Autodesk Inventor part; units mm, degrees
ref_plane "Work Plane1" through (0, 0, 4950) normal (0, 0, 1) x (1, 0, 0)
ref_plane "Work Plane2" through (0, 0, 4954) normal (0, 0, 1) x (1, 0, 0)
ref_plane "Work Plane3" through (-40, 73, 4950) normal (0, -1, 0) x (1, 0, 0)
ref_plane "Work Plane1" through (0, 0, 4950) normal (0, 0, 1) x (1, 0, 0)
sketch "Sketch1" plane through (0, 0, 4950) normal (0, 0, 1) x (1, 0, 0)
  circle A0 centre (180, 0) radius 12.5
  circle A1 centre (180, 17.5) radius 2
  circle A2 centre (197.5, 0) radius 2
  circle A3 centre (162.5, 0) radius 2
  circle A4 centre (180, -17.5) radius 2
  line L0 (40, 182.7) -> (-40, 182.7)
  line L1 (-40, 182.7) -> (-40, -182.7)
  line L2 (-40, -182.7) -> (40, -182.7)
  line L3 (40, -182.7) -> (40, -50)
  line L4 (40, -50) -> (260, -50)
  line L5 (260, -50) -> (260, 50)
  line L6 (260, 50) -> (40, 50)
  line L7 (40, 50) -> (40, 182.7)
  circle A5 centre (0, 120) radius 8
  circle A6 centre (0, -120) radius 8
  circle A7 centre (0, -120) radius 8.5
  circle A8 centre (0, 120) radius 8.5
  line L8 (40, 182.7) -> (40, -182.7)
  line L9 (40, -182.7) -> (80, -182.7)
  line L10 (80, -182.7) -> (80, 182.7)
  line L11 (80, 182.7) -> (40, 182.7)
  line L12 (-40, 75) -> (40, 75)
  line L13 (40, 75) -> (40, -75)
  line L14 (40, -75) -> (-40, -75)
  line L15 (80, 182.7) -> (260, 50)
  line L16 (260, -50) -> (80, -182.7)
  line L17 (80, -142.7) -> (-40, -142.7)
  line L18 (-40, 142.7) -> (80, 142.7)
  line L19 (80, 142.7) -> (134.2577, 142.7)
  line L20 (80, -142.7) -> (134.2577, -142.7)
  line L21 (210, 86.8611) -> (210, -86.8611)
  point P0 (0, 0)
  point P1 (40, 75)
  dimension "d0" = 17
  dimension "d1" = 17
  dimension "d2" = 40
  dimension "d3" = 40
  dimension "d4" = 75
  dimension "d5" = 75
  dimension "d23" = 40
  dimension "d24" = 40
  dimension "d25" = 50
extrude "Extrusion1" add sketch "Sketch1" along normal blind 8 contours A0 | A1 | A2 | A3 | A4 | L18 L10 L6 L7 | L7 L12 L1 L18 | L19 L15 L21 L6 L10 | L6 L10 L4 L8 | L6 L21 L4 L10 | L14 L3 L17 L1 | L4 L10 L17 L3 | L4 L21 L16 L20 L10
sketch "Sketch2" plane through (0, 0, 4958) normal (0, 0, 1) x (1, 0, 0)
  line L0 (-40, 75) -> (40, 75)
  line L1 (-40, 75) -> (40, 75)
  line L2 (40, 75) -> (40, 79)
  line L3 (40, 79) -> (-40, 79)
  line L4 (-40, 79) -> (-40, 75)
  line L5 (40, -75) -> (-40, -75)
  line L6 (40, -75) -> (-40, -75)
  line L7 (-40, -75) -> (-40, -79)
  line L8 (-40, -79) -> (40, -79)
  line L9 (40, -79) -> (40, -75)
  line L10 (-20, 79) -> (-20, -79)
  line L11 (20, -79) -> (20, 79)
  point P0 (0, 0)
  point P1 (20, 75)
  point P2 (-20, 75)
  point P3 (20, -75)
  point P4 (-20, -75)
  dimension "d8" = 4
  dimension "d9" = 4
  dimension "d12" = 20
  dimension "d13" = 20
extrude "Extrusion2" add sketch "Sketch2" along normal blind 50 contours L10 L3 L11 L0 | L5 L11 L8 L10
sketch "Sketch3" plane through (-40, -75, 4950) normal (0, 1, 0) x (1, 0, 0)
  circle A0 centre (40, -38) radius 10.5
  line L0 (60, -58) -> (20, -58)
  line L1 (20, -8) -> (20, -58)
  point P0 (40, 4950)
  dimension "d16" = 21
  dimension "d17" = 20
  dimension "d18" = 20
extrude "Extrusion3" add sketch "Sketch3" along normal blind 163 and the other way blind 13
sketch "Sketch4" plane through (0, 0, 4958) normal (0, 0, 1) x (1, 0, 0)
  circle A0 centre (160, 17.5) radius 2
  circle A1 centre (177.5, 0) radius 2
  circle A2 centre (0, -120) radius 8
  circle A3 centre (142.5, 0) radius 2
  circle A4 centre (160, -17.5) radius 2
  circle A5 centre (0, 120) radius 8
  line L0 (30, 157.3) -> (30, 182.7)
  line L1 (40, 182.7) -> (30, 182.7)
  line L2 (40, 50) -> (40, 182.7)
  line L3 (260, 50) -> (40, 50)
  line L4 (260, -50) -> (260, 50)
  line L5 (40, -50) -> (260, -50)
  line L6 (40, -182.7) -> (40, -50)
  line L7 (30, -182.7) -> (40, -182.7)
  line L8 (30, -182.7) -> (30, -157.3)
  line L9 (30, -157.3) -> (-30, -157.3)
  line L10 (-30, -157.3) -> (-30, -182.7)
  line L11 (-40, -182.7) -> (-30, -182.7)
  line L12 (-40, 182.7) -> (-40, -182.7)
  line L13 (-30, 182.7) -> (-40, 182.7)
  line L14 (-30, 182.7) -> (-30, 157.3)
  line L15 (-30, 157.3) -> (30, 157.3)
  line L16 (250, 25.4) -> (224.6, 25.4)
  line L17 (224.6, 25.4) -> (224.6, -25.4)
  line L18 (224.6, -25.4) -> (250, -25.4)
  line L19 (250, -25.4) -> (250, 25.4)
  circle A6 centre (160, 0) radius 10
  point P0 (0, 0)
extrude "Extrusion4" cut sketch "Sketch4" against normal up to surface (8 mm away) contours A0 | A1 | A3 | A4
sketch "Sketch5" plane through (0, 0, 4958) normal (0, 0, 1) x (1, 0, 0)
  circle A0 centre (160, 0) radius 7.5
  circle A1 centre (160, 0) radius 8.25
  point P0 (0, 0)
  dimension "d28" = 16.5
extrude "Extrusion5" cut sketch "Sketch5" against normal blind 10 contours A0 | A1
sketch "Sketch6" plane through (0, 0, 4950) normal (0, 0, -1) x (-1, 0, 0)
  circle A0 centre (-142.5, 0) radius 2
  circle A1 centre (-177.5, 0) radius 2
  circle A2 centre (-160, 17.5) radius 2
  circle A3 centre (-160, -17.5) radius 2
  line L0 (-134.2577, 142.7) -> (40, 142.7)
  line L1 (-210, 86.8611) -> (-134.2577, 142.7)
  line L2 (-210, -86.8611) -> (-210, 86.8611)
  line L3 (-134.2577, -142.7) -> (-210, -86.8611)
  line L4 (40, -142.7) -> (-134.2577, -142.7)
  line L5 (40, -75) -> (40, -142.7)
  line L6 (-40, -75) -> (40, -75)
  line L7 (-40, 75) -> (-40, -75)
  line L8 (40, 75) -> (-40, 75)
  line L9 (40, 142.7) -> (40, 75)
  circle A4 centre (0, -120) radius 8.5
  circle A5 centre (0, 120) radius 8.5
  circle A6 centre (-160, 0) radius 8.25
  circle A7 centre (-160, 0) radius 22.5
  point P0 (0, 0)
  dimension "d31" = 45
extrude "Extrusion6" add sketch "Sketch6" along normal blind 4 contours A7
sketch "Sketch7" plane through (160, 0, 4946) normal (0, 0, -1) x (-1, 0, 0)
  circle A0 centre (0, 0) radius 22.5
  circle A1 centre (0, 0) radius 12.5
  circle A2 centre (0, 0) radius 9
  point P0 (160, 0)
  dimension "d34" = 25
  dimension "d47" = 18
extrude "Extrusion7" add sketch "Sketch7" along normal blind 40 contours A1
sketch "Sketch9" plane through (0, 0, 5008) normal (0, 0, 1) x (1, 0, 0)
  circle A0 centre (160, 0) radius 8.25 construction
  circle A1 centre (142.5, 0) radius 2 construction
  circle A2 centre (177.5, 0) radius 2 construction
  circle A3 centre (160, 17.5) radius 2 construction
  circle A4 centre (160, -17.5) radius 2 construction
  line L0 (20, 79) -> (20, 75)
  line L1 (20, 75) -> (40, 75)
  line L2 (40, 75) -> (40, -75)
  line L3 (40, -75) -> (20, -75)
  line L4 (20, -75) -> (20, -79)
  line L5 (20, -79) -> (-20, -79)
  line L6 (-20, -79) -> (-20, -75)
  line L7 (-20, -75) -> (-40, -75)
  line L8 (-40, -75) -> (-40, -142.7)
  line L9 (-40, -142.7) -> (134.2577, -142.7)
  line L10 (134.2577, -142.7) -> (210, -86.8611)
  line L11 (210, -86.8611) -> (210, 86.8611)
  line L12 (210, 86.8611) -> (134.2577, 142.7)
  line L13 (134.2577, 142.7) -> (-40, 142.7)
  line L14 (-40, 142.7) -> (-40, 75)
  line L15 (-40, 75) -> (-20, 75)
  line L16 (-20, 75) -> (-20, 79)
  line L17 (-20, 79) -> (20, 79)
  circle A5 centre (0, -120) radius 8.5
  circle A6 centre (0, 120) radius 8.5
  circle A7 centre (160, 0) radius 12.5
  circle A8 centre (160, 0) radius 9
  line L18 (20, -75) -> (-20, -75)
  line L19 (-20, 75) -> (20, 75)
  point P0 (0, 0)
  dimension "d37" = 18
extrude "Extrusion8" [suppressed]
sketch "Sketch10" plane through (0, 0, 5012) normal (0, 0, 1) x (1, 0, 0)
  circle A0 centre (120, -75) radius 6
  circle A1 centre (90, 0) radius 6
  circle A2 centre (120, 75) radius 6
  circle A3 centre (160, 0) radius 12.5
  point P0 (0, 0)
  dimension "d40" = 70
  dimension "d41" = 75
  dimension "d42" = 75
  dimension "d43" = 40
  dimension "d44" = 12
extrude "Extrusion9" [suppressed]
sketch "Sketch11" plane through (20, -79, 4958) normal (1, 0, 0) x (0, 0, -1)
  line L0 (0, 4) -> (0, 0)
  line L1 (0, 4) -> (-50, 4)
  line L2 (-50, 0) -> (-50, 4)
  line L3 (0, 0) -> (-50, 0)
  line L4 (0, 158) -> (0, 154)
  line L5 (0, 158) -> (-50, 158)
  line L6 (-50, 154) -> (-50, 158)
  line L7 (0, 154) -> (-50, 154)
  point P0 (4958, 79)
extrude "Extrusion10" add sketch "Sketch11" along normal blind 190
sketch "Sketch12" plane through (-20, -79, 4958) normal (-1, 0, 0) x (0, 0, 1)
  line L0 (0, 154) -> (0, 158)
  line L1 (0, 154) -> (50, 154)
  line L2 (50, 158) -> (50, 154)
  line L3 (0, 158) -> (50, 158)
  line L4 (0, 0) -> (0, 4)
  line L5 (0, 0) -> (50, 0)
  line L6 (50, 4) -> (50, 0)
  line L7 (0, 4) -> (50, 4)
  point P0 (-4958, 79)
extrude "Extrusion11" add sketch "Sketch12" along normal up to surface (20 mm away)
ref_plane "Work Plane2" through (0, 0, 4954) normal (0, 0, 1) x (1, 0, 0)
mirror "Mirror1" about plane through (0, 0, 4954) normal (0, 0, 1) of "Extrusion6", "Extrusion7"
sketch "Sketch13" plane through (160, 0, 4906) normal (0, 0, -1) x (-1, 0, 0)
  circle A0 centre (0, 0) radius 9
  circle A1 centre (4, 28) radius 75.6042
  point P0 (160, 0)
extrude "Extrusion12" cut sketch "Sketch13" against normal up to surface (44 mm away)
ref_plane "Work Plane3" through (-40, 73, 4950) normal (0, -1, 0) x (1, 0, 0)
sketch "Sketch14" plane through (-40, 73, 4950) normal (0, -1, 0) x (1, 0, 0)
  circle A0 centre (40, 38) radius 10.5
  line L0 (0, 8) -> (250, 8)
  line L1 (0, 8) -> (0, 58)
  line L2 (0, 58) -> (250, 58)
  line L3 (250, 8) -> (250, 58)
  circle A1 centre (40, 38) radius 12
  point P0 (40, -4950)
  dimension "d55" = 24
extrude "Extrusion13" add sketch "Sketch14" along normal blind 2 contours A1
mirror "Mirror2" about plane through (0, 0, 0) normal (0, 1, 0) of "Extrusion13"
ref_plane "Work Plane4" through (-40, 0, 4950) normal (0, 1, 0) x (1, 0, 0)
sketch "Sketch15" plane through (-40, 0, 4950) normal (0, 1, 0) x (1, 0, 0)
  circle A0 centre (40, -38) radius 10.5
  circle A1 centre (40, -38) radius 10.5
  circle A2 centre (40, -38) radius 17.5
  point P0 (40, 4950)
  dimension "d58" = 35
extrude "Extrusion14" add sketch "Sketch15" along normal mid plane 37
pattern_linear "Rectangular Pattern1" count 2 spacing 29 along (0, -1, 0) of "Extrusion13"
mirror "Mirror3" about plane through (0, 0, 0) normal (0, 1, 0) of "Extrusion13", "Rectangular Pattern1"
equation "\"d8\" = d9"
properties part number "base for ball scew -bolt" material "Steel, Mild"
Geometry check sheet. Reference: the model listing, model coordinates, mm. A direction names the side the tool comes from. Round coordinates to 2 decimals unless told otherwise and drop trailing zeros. Loops run counter-clockwise (first coordinate to the right, second up) from the corner with the lowest first, then second, coordinate; pieces in that order, holes last. Notation, with made-up numbers: (3.5, -2) - (18.5, -2) arc R20 cw to (18.5, 20) - close; hole circle Ø2 at (24, 62.25). An arc over 180 degrees is marked (long way). Use a Markdown table: item, result.
Q1. Cross-section at C-C on x = 85. Record the cut outline in (y, z), plus the area to 3 significant figures.
Solutions:
| item | result |
|---|---|
| outline | (-142.7, 4950) - (142.7, 4950) - (142.7, 4958) - (79, 4958) - (79, 5008) - (75, 5008) - (75, 4958) - (-75, 4958) - (-75, 5008) - (-79, 5008) - (-79, 4958) - (-142.7, 4958) - close |
| area | 2,680 mm2 |
Q2. Access from +Z, -Z, +X, -X, +Y, -Y to the whole of each face (thin tool, end or side, straight path). Record for faces 4 (the flat face through (0, -88, 4988)), 5 (the flat face through (163, -8, 4962)), 6 (the cylindrical face through (169, 0, 4948)), 7 (the flat face through (0, 71, 4977)).
Solutions:
| item | result |
|---|---|
| face 4 | +Z, +X, -X, -Y |
| face 5 | +Z |
| face 6 | -Z |
| face 7 | none |
Q3. Cross-section at A-A on y = 120. Record the cut outline in (x, z), plus the area to 3 significant figures.
Solutions:
| item | result |
|---|---|
| outline | (-40, 4950) - (-8.5, 4950) - (-8.5, 4958) - (-40, 4958) - close; (8.5, 4950) - (165.05, 4950) - (165.05, 4958) - (8.5, 4958) - close |
| area | 1,500 mm2 |
Q4. Go/stop test with flat-tipped pins: P1, Ø8, axis at y = -43, z = 5000.5, coming from the -X side; P2, Ø19, axis at x = 160, y = 0, coming from the +Z side; P3, Ø8, axis at x = 3.5, z = 4974.5, coming from the -Y side. Record where each tip stops, or that it passes through.
Solutions:
| item | result |
|---|---|
| P1 | stops at x = -8.47 |
| P2 | stops at z = 5002 |
| P3 | stops at y = -88 |
Q5. Material ranges on line 1 (Y direction, x = 160, z = 4959.45); line 2 (Y direction, x = 160, z = 4952.25); line 3 (Y direction, x = 188, z = 4992.5), recorded low to high.
Solutions:
| item | result |
|---|---|
| line 1 | y = -79 to -75, -22.5 to -19.5, -15.5 to -8.25, 8.25 to 15.5, 19.5 to 22.5, 75 to 79 |
| line 2 | y = -123.72 to -19.5, -15.5 to -8.25, 8.25 to 15.5, 19.5 to 123.72 |
| line 3 | y = -79 to -75, 75 to 79 |
Q6. Draft check along Y on faces 1 (the flat face through (83, 111, 4958)), 2 (the cylindrical face through (-2.28, 57.31, 4977.75)), 3 (the flat face through (171.6, 115.17, 4953.94)). Enter one of: released by +Y, released by -Y, zero draft, split by the parting line, or undercut.
Solutions:
| item | result |
|---|---|
| face 1 | zero draft |
| face 2 | undercut |
| face 3 | released by +Y |
Q7. Cross-section at B-B on z = 4988. State how many separate pieces and enclosed holes the cut face has, plus the area to 3 significant figures.
Solutions:
| item | result |
|---|---|
| separate pieces | 2 |
| enclosed holes | 1 |
| area | 6,310 mm2 |
Q8. Cross-section at D-D on y = 82.5. Record the cut outline in (x, z).
Solutions:
| item | result |
|---|---|
| outline | (-40, 4950) - (210, 4950) - (210, 4958) - (-40, 4958) - close; circle Ø21 at (0, 4988) |
